Verification items for the finished model (mm, model axes). Give positions to 0.01 mm unless a question says otherwise; leave off trailing zeros. Write each loop counter-clockwise with the first axis right and the second up, starting at its lowest first coordinate (ties: lowest second). Pieces come first, ordered by that corner, then holes.
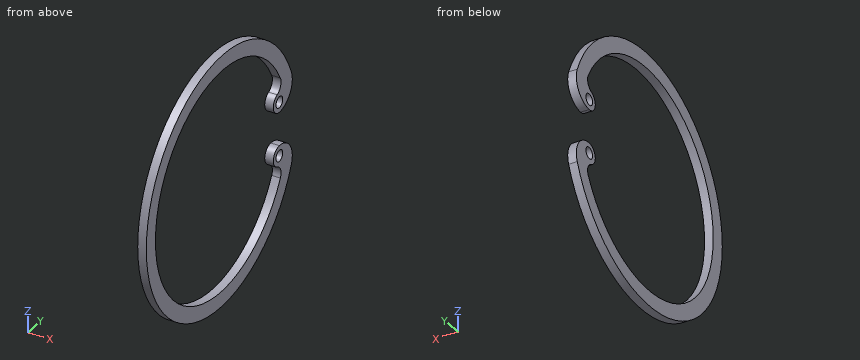
from build123d import *

# Parameters (mm, degrees)
SKETCH_1_R      = 1.25
EXTRUDE_1_DEPTH = 1.9


with BuildPart() as part:
    # Эскиз1 → Бобышка-Вытянуть1 (new body)
    with BuildSketch(Plane(origin=(0, 0, 0), x_dir=(0, 0, -1), z_dir=(1, 0, 0))):
        with BuildLine():
            ThreePointArc((-10.357624838, 26.121439618), (0, -28.1), (10.357624838, 26.121439618))
            ThreePointArc((10.357624838, 26.121439618), (5.865289545, 25.627220585), (3.75, 21.633365434))
            ThreePointArc((3.75, 21.633365434), (5.585080517, 19.421953708), (8.096970509, 20.817758491))
            ThreePointArc((8.096970509, 20.817758491), (9.392356028, 22.104521997), (11.215605485, 22.006821525))
            ThreePointArc((11.215605485, 22.006821525), (0, -24.7), (-11.215605485, 22.006821525))
            ThreePointArc((-11.215605485, 22.006821525), (-9.392356028, 22.104521997), (-8.096970509, 20.817758491))
            ThreePointArc((-8.096970509, 20.817758491), (-5.585080517, 19.421953708), (-3.75, 21.633365434))
            ThreePointArc((-3.75, 21.633365434), (-5.865289545, 25.627220585), (-10.357624838, 26.121439618))
        make_face()
        with Locations((-6, 21.633365434)):
            Circle(SKETCH_1_R, mode=Mode.SUBTRACT)
        with Locations((6, 21.633365434)):
            Circle(SKETCH_1_R, mode=Mode.SUBTRACT)
    extrude(amount=EXTRUDE_1_DEPTH)


solid = part.part
Item 1: Sectioned sample at D-D on z = 6. Record the cut outline in (x, y).
Answer key:
outline: (0, -27.45) - (1.9, -27.45) - (1.9, -23.96) - (0, -23.96) - close; (0, 19.38) - (1.9, 19.38) - (1.9, 20.38) - (0, 20.38) - close; (0, 22.88) - (1.9, 22.88) - (1.9, 25.72) - (0, 25.72) - close
Item 2: Scan lines: line 1 along Y through (x, z) = (1.35, -6); line 2 along Z through (x, y) = (0.9, 0); line 3 along Y through (x, z) = (1.5, 0). Record each from-to range of solid material in increasing order.
Answer key:
line 1: y = -27.45 to -23.96, 19.38 to 20.38, 22.88 to 25.72
line 2: z = -28.1 to -24.7, 24.7 to 28.1
line 3: y = -28.1 to -24.7
Item 3: Sectioned sample at A-A on x = 1.4. Record the cut outline in (y, z), then the cut area to 3 significant figures.
Answer key:
outline: (20.82, -8.1) arc R2.25 cw to (22.01, -11.22) arc R24.7 cw (long way) to (22.01, 11.22) arc R2.25 cw to (20.82, 8.1) arc R2.25 ccw to (21.63, 3.75) arc R4.83 ccw to (26.12, 10.36) arc R28.1 ccw (long way) to (26.12, -10.36) arc R4.83 ccw to (21.63, -3.75) arc R2.25 ccw to start; hole circle Ø2.5 at (21.63, -6); hole circle Ø2.5 at (21.63, 6)
area: 550 mm2
Item 4: Sectioned sample at B-B on y = -3. Record the cut outline in (x, z).
Answer key:
outline: (0, -27.94) - (1.9, -27.94) - (1.9, -24.52) - (0, -24.52) - close; (0, 24.52) - (1.9, 24.52) - (1.9, 27.94) - (0, 27.94) - close
Item 5: Sectioned sample at C-C on z = 18. Record the cut outline in (x, y), then the cut area to 3 significant figures.
Answer key:
outline: (0, -21.58) - (1.9, -21.58) - (1.9, -16.91) - (0, -16.91) - close; (0, 16.91) - (1.9, 16.91) - (1.9, 21.58) - (0, 21.58) - close
area: 17.7 mm2
